Geometry: final body of the model. Coordinates: model frame, mm. Face numbers are marked on the shaded views. A direction names the side the tool comes from. Round coordinates to 2 decimals unless told otherwise and drop trailing zeros. Loops run counter-clockwise (first coordinate to the right, second up) from the corner with the lowest first, then second, coordinate; pieces in that order, holes last. Notation, with made-up numbers: (-11, 63.25) - (4, 63.25) arc R6 ccw to (4, 74.25) - close; hole circle Ø9 at (40, 11). An arc over 180 degrees is marked (long way). Return JSON: item names as keys, results as strings. Group by question number.
1. Section C-C on z = 0. Return loops of the section in (x, y), and give its area (3 significant figures).
2. Section A-A on x = 0. Return loops of the section in (y, z).
3. Draft query along Z for the marked faces 1, 2 and 3. Return one class per face: +Z half, -Z half, draft (parallel to the pull), parting line (faces both ways), or undercut.
4. Section B-B on y = 0.5. Return loops of the section in (x, z).
5. First-contact query: pin 1 Ø3 at (y, z) = (2.5, 5.5) entering from -X; pin 2 Ø4 at (x, z) = (0, 0) entering from +Y; pin 3 Ø3.5 at (x, z) = (0, 0) entering from -Y; pin 4 Ø4.5 at (x, z) = (-1, 0) entering from +Y. Flat tips, straight axial feed; report the tip coordinate or a pass-through.
6. Material intervals for probe 1 along Z at (x, y) = (0, 5.35); probe 2 along Y at (x, z) = (8, -5.5); probe 3 along Z at (x, y) = (8, 3.7), sorted ascending.
7. Section D-D on z = 8. Return loops of the section in (x, y), and give its area (3 significant figures).
8. Set-up query: the marked faces 4, 5 and 6. Return all of +Z, -Z, +X, -X, +Y, -Y with unobstructed straight access to the full face (end or side cutting, diameter ignored); none if empty.
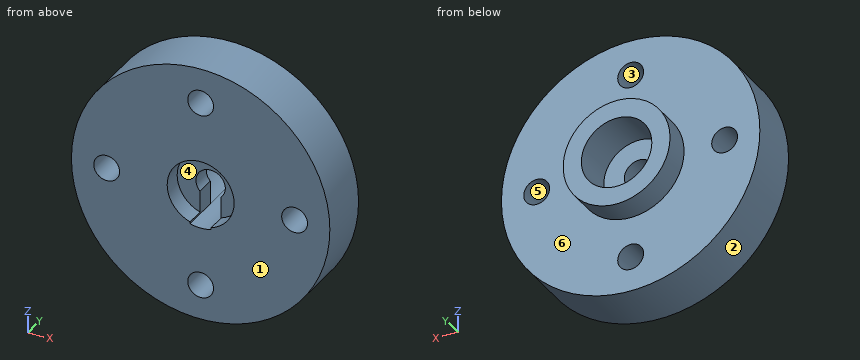
from build123d import *

# Parameters (mm, degrees)
CUT_EXTRUDE1_DEPTH      = 16.967466925
CUT_EXTRUDE1_DEPTH_BACK = 16.967466925
SKETCH5_R               = 1.1
CUT_EXTRUDE2_DEPTH      = 10


with BuildPart() as part:
    # Sketch3 → Revolve1 (revolve)
    with BuildSketch(Plane.XY, mode=Mode.PRIVATE) as revolve1_sk:
        Polygon((2.85, 0), (11, 0), (11, 4.6), (4.55, 4.6), (4.55, 6.85), (3, 6.85), (3, 3.25), (0, 3.25), (0, 1.6), (2.85, 1.6), align=None)
    revolve(revolve1_sk.sketch.rotate(Axis((0, 3.25, 0), (0, -1, 0)), 180), axis=Axis((0, 3.25, 0), (0, -1, 0)))

    # Sketch4 → Cut-Extrude1 (cut, two sides: drawn at the far end of the back side and taken through both)
    with BuildSketch(Plane(origin=(0, 3.25, 0), x_dir=(1, 0, 0), z_dir=(0, 1, 0)).offset(-CUT_EXTRUDE1_DEPTH_BACK)):
        with BuildLine():
            Line((-0.9, 2.861817604), (-0.9, 0.867467579))
            ThreePointArc((-0.9, 0.867467579), (0, -1.25), (0.9, 0.867467579))
            Line((0.9, 0.867467579), (0.9, 2.861817604))
            ThreePointArc((0.9, 2.861817604), (0, 3), (-0.9, 2.861817604))
        make_face()
    extrude(amount=CUT_EXTRUDE1_DEPTH + CUT_EXTRUDE1_DEPTH_BACK, mode=Mode.SUBTRACT)

    # Sketch5 → Cut-Extrude2 (cut)
    with BuildSketch(Plane.XZ):
        with Locations((0, 8)):
            Circle(SKETCH5_R)
        with Locations((8, 0)):
            Circle(SKETCH5_R)
        with Locations((0, -8)):
            Circle(SKETCH5_R)
        with Locations((-8, 0)):
            Circle(SKETCH5_R)
    extrude(amount=-CUT_EXTRUDE2_DEPTH, mode=Mode.SUBTRACT)


solid = part.part
Taken from the geometry:
{
 "1": {"outline": "(-11, 0) - (-9.1, 0) - (-9.1, 4.6) - (-11, 4.6) - close; (-6.9, 0) - (-2.85, 0) - (-2.85, 1.6) - (-1.25, 1.6) - (-1.25, 3.25) - (-3, 3.25) - (-3, 6.85) - (-4.55, 6.85) - (-4.55, 4.6) - (-6.9, 4.6) - close; (1.25, 1.6) - (2.85, 1.6) - (2.85, 0) - (6.9, 0) - (6.9, 4.6) - (4.55, 4.6) - (4.55, 6.85) - (3, 6.85) - (3, 3.25) - (1.25, 3.25) - close; (9.1, 0) - (11, 0) - (11, 4.6) - (9.1, 4.6) - close", "area": "66.6 mm2"},
 "2": {"outline": "(0, -11) - (4.6, -11) - (4.6, -9.1) - (0, -9.1) - close; (0, -6.9) - (4.6, -6.9) - (4.6, -4.55) - (6.85, -4.55) - (6.85, -3) - (0, -3) - close; (0, 2.85) - (1.6, 2.85) - (1.6, 1.25) - (3.25, 1.25) - (3.25, 3) - (6.85, 3) - (6.85, 4.55) - (4.6, 4.55) - (4.6, 6.9) - (0, 6.9) - close; (0, 9.1) - (4.6, 9.1) - (4.6, 11) - (0, 11) - close"},
 "3": {"face 1": "draft", "face 2": "parting line", "face 3": "undercut"},
 "4": {"outline": "circle Ø22 at (0, 0); hole circle Ø2.2 at (-8, 0); hole circle Ø2.2 at (0, -8); hole circle Ø2.2 at (0, 8); hole (-0.9, -2.86) arc R3 ccw to (0.9, -2.86) - (0.9, -2.7) arc R2.85 ccw (long way) to (-0.9, -2.7) - close; hole circle Ø2.2 at (8, 0)"},
 "5": {"pin 1": "x = -10.25", "pin 2": "y = 3.25", "pin 3": "y = 1.6", "pin 4": "y = 6.85"},
 "6": {"probe 1": "-4.55 to -3, 3 to 4.55", "probe 2": "0 to 4.6", "probe 3": "-7.55 to -1.1, 1.1 to 7.55"},
 "7": {"outline": "(-7.55, 0) - (-1.1, 0) - (-1.1, 4.6) - (-7.55, 4.6) - close; (1.1, 0) - (7.55, 0) - (7.55, 4.6) - (1.1, 4.6) - close", "area": "59.3 mm2"},
 "8": {"face 4": "-Y", "face 5": "+Y, -Y", "face 6": "+Y"}
}
